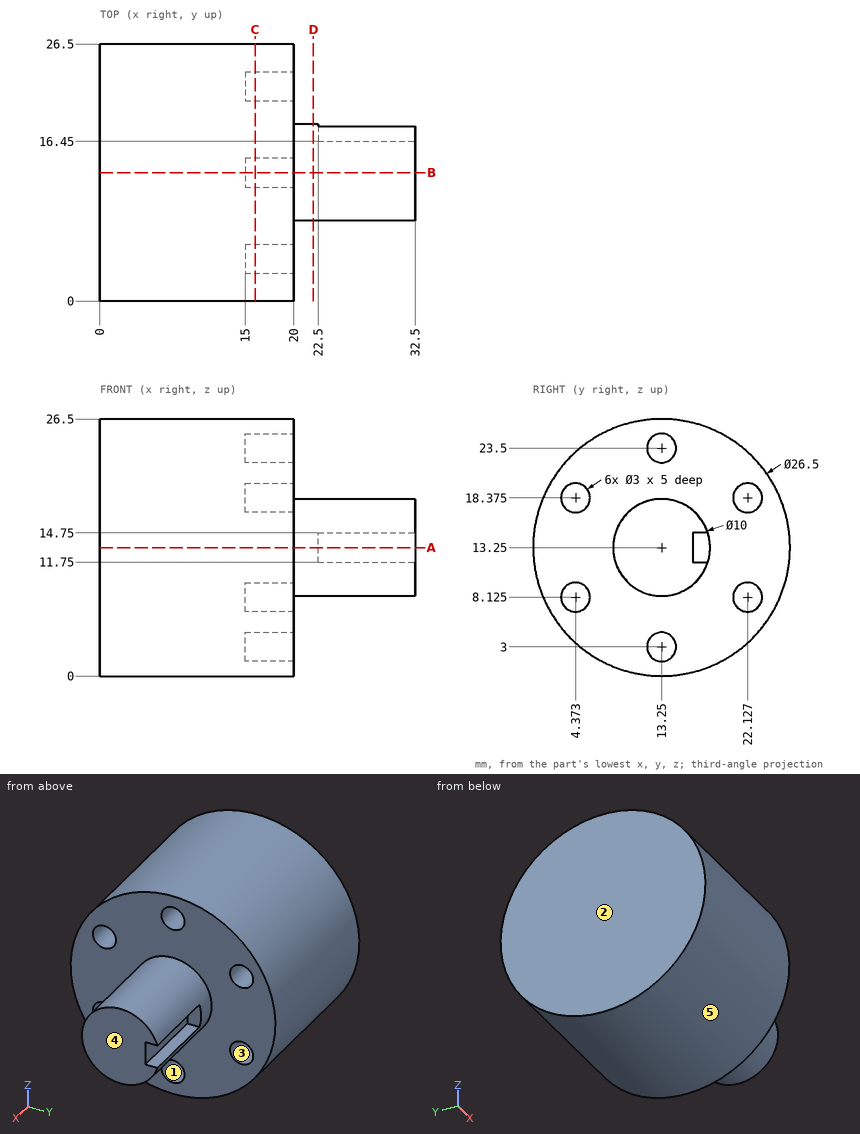
For this review, use the dimensioned drawing (mm, ordinates from the lowest corner) and the shaded views. A direction names the side the tool comes from. Coordinates: 2 decimals unless noted, no trailing zeros. Order: outer loops, then holes, each group sorted by start corner. A loop starts at its lowest first (then second) coordinate and runs counter-clockwise, first axis right, second up. Notation, with made-up numbers: (-9, 76) -> (27, 76) arc R35 ccw to (27, 114) -> close; hole circle Ø10 at (42.25, -21). An arc over 180 degrees is marked (long way). One line per item, written item: value. Start each with the question number.
Q1. For probe 1 along X at (y, z) = (9, 5); probe 2 along Y at (x, z) = (18.5, 9) (1 decimal); probe 3 along Y at (x, z) = (18, 8.75), list the stretches that pass through material, from the lowest coordinate up.
Q2. Take a section at B-B, the plane y = 13.25. State the section outline as (x, z) points.
Q3. Take a section at C-C, the plane x = 16. Give the number of separate pieces and of enclosed holes in the cut face, then the cut area to 3 significant figures.
Q4. Mouldability with a two-part tool opening along Z and no side actions: class the marked faces 3, 4 and 5 as pulls with the +Z half, pulls with the -Z half, needs draft (parallel to the pull), parting line crosses it, or undercut.
Q5. Take a section at A-A, the plane z = 13.25. State the section outline as (x, y) points.
Q6. Take a section at D-D, the plane x = 22. State the section outline as (y, z) points.
Q7. Insertion check: pin 1 Ø0.9 at (y, z) = (13.5, 23) entering from +X; pin 2 Ø1.5 at (x, z) = (29.5, 13.5) entering from +Y; pin 3 Ø1 at (x, z) = (6, 3.5) entering from -Y; pin 4 Ø3.5 at (y, z) = (4.37, 8.12) entering from -X. Each pin has a flat end and moves straight along its axis. Give the tip position at first contact, or say it passes through.
Q8. Tool access review of the marked faces 1 and 2: name each direction out of +Z, -Z, +X, -X, +Y, -Y from which nothing blocks a thin tool from reaching the whole face with its end or side.
Values follow:
1. probe 1: x = 0 to 20
1. probe 2: y = 0.7 to 3.2, 5.6 to 20.9, 23.3 to 25.8
1. probe 3: y = 0.79 to 3.01, 5.74 to 20.76, 23.49 to 25.71
2. outline: (0, 0) -> (20, 0) -> (20, 1.5) -> (15, 1.5) -> (15, 4.5) -> (20, 4.5) -> (20, 8.25) -> (32.5, 8.25) -> (32.5, 18.25) -> (20, 18.25) -> (20, 22) -> (15, 22) -> (15, 25) -> (20, 25) -> (20, 26.5) -> (0, 26.5) -> close
3. separate pieces: 1
3. enclosed holes: 6
3. area: 509 mm2
4. face 3: undercut
4. face 4: needs draft
4. face 5: parting line crosses it
5. outline: (0, 0) -> (20, 0) -> (20, 8.25) -> (32.5, 8.25) -> (32.5, 16.45) -> (22.5, 16.45) -> (22.5, 18.25) -> (20, 18.25) -> (20, 26.5) -> (0, 26.5) -> close
6. outline: circle Ø10 at (13.25, 13.25)
7. pin 1: stops at x = 15
7. pin 2: stops at y = 16.45
7. pin 3: stops at y = 3.76
7. pin 4: stops at x = 0
8. face 1: +X
8. face 2: +Z, -Z, -X, +Y, -Y
